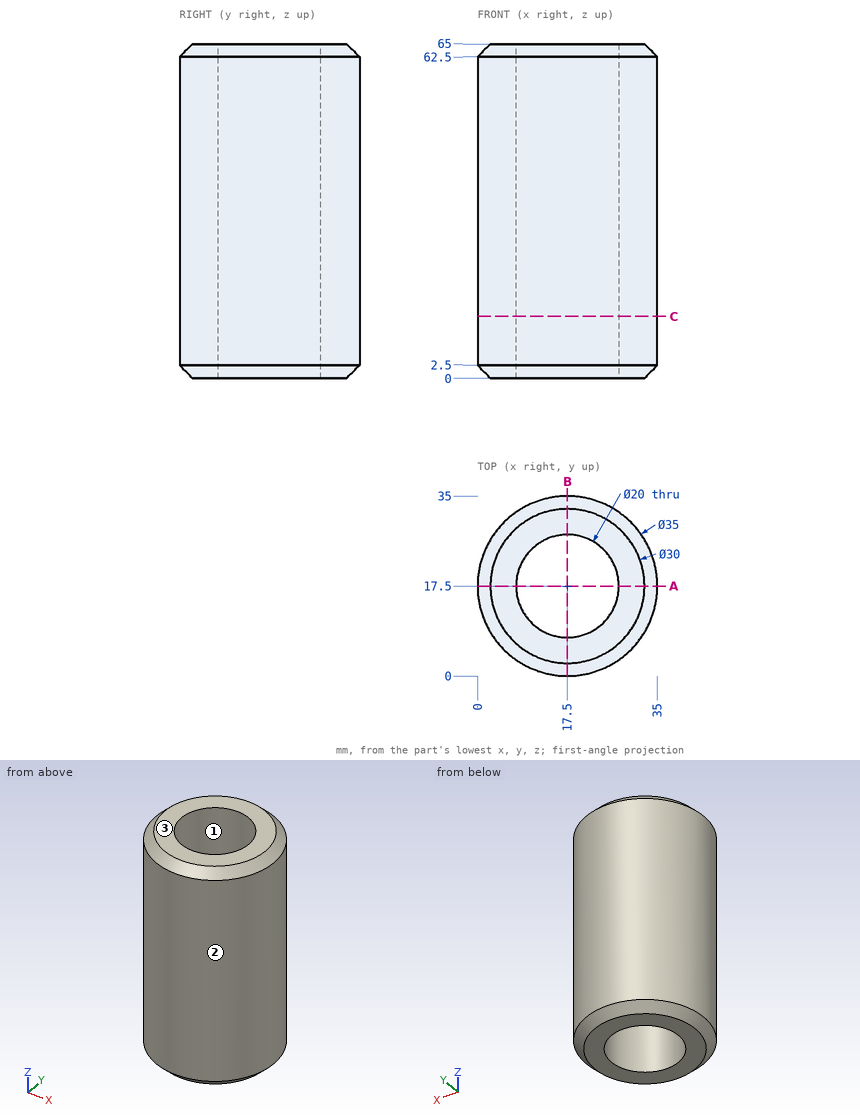
Verification items for this drawing (mm, ordinates from the low corner). Coordinates: 2 decimals unless noted, no trailing zeros. Write each loop counter-clockwise with the first axis right and the second up, starting at its lowest first coordinate (ties: lowest second). Pieces come first, ordered by that corner, then holes. Notation, with made-up numbers: (40.5, 72) - (45.5, 72) arc R15 cw to (45.5, 78) - close; hole circle Ø2 at (-24.5, 32). An arc over 180 degrees is marked (long way). One line per question, with ' | ' between items.
Item 1: Mould release check, pull along Y, two halves, no side actions. Record for the marked faces 1, 2 and 3: pulls with the +Y half, pulls with the -Y half, needs draft (parallel to the pull), parting line crosses it, or undercut.
Determined:
face 1: undercut | face 2: parting line crosses it | face 3: needs draft
Item 2: Sectioned sample at A-A on y = 17.5. Record the boundary of the cut face in (x, z), plus the area to 4 significant figures.
Determined:
outline: (0, 2.5) - (2.5, 0) - (7.5, 0) - (7.5, 65) - (2.5, 65) - (0, 62.5) - close; (27.5, 0) - (32.5, 0) - (35, 2.5) - (35, 62.5) - (32.5, 65) - (27.5, 65) - close | area: 962.5 mm2
Item 3: Thickness scan on line 1 (X direction, y = 17, z = 40); line 2 (Y direction, x = 17.5, z = 50); line 3 (X direction, y = 19, z = 52.5). Record the ranges inside material, lowest first. Write a range as [from, to].
Determined:
line 1: x = [0.01, 7.51], [27.49, 34.99] | line 2: y = [0, 7.5], [27.5, 35] | line 3: x = [0.06, 7.61], [27.39, 34.94]
Item 4: Gauge pin test, flat ends, axial feed: P1, Ø1, axis at y = 19.5, z = 12, coming from the +X side; P2, Ø1.5, axis at x = 14, z = 50, coming from the -Y side; P3, Ø4, axis at y = 10.5, z = 51, coming from the +X side. Record the tip position at first contact, or that the pin passes through.
Determined:
P1: stops at x = 34.94 | P2: stops at y = 0.22 | P3: stops at x = 34.27
Item 5: Sectioned sample at C-C on z = 12. Record the boundary of the cut face in (x, y).
Determined:
outline: circle Ø35 at (17.5, 17.5); hole circle Ø20 at (17.5, 17.5)
